```python
from build123d import *

# Parameters (mm, degrees)
CROQUIS1_W               = 70
CROQUIS1_H               = 64.6
CROQUIS1_W_2             = 50
CROQUIS1_H_2             = 44.6
SALIENTE_EXTRUIR1_DEPTH  = 5
CROQUIS2_W               = 8
CROQUIS2_H               = 5
SALIENTE_EXTRUIR2_DEPTH  = 5
REDONDEO1_R              = 0.5
REDONDEO1_OF_SIMETR_A1_R = 0.5
REDONDEO2_R              = 5


with BuildPart() as part:
    # Croquis1 → Saliente-Extruir1 (new body)
    with BuildSketch(Plane.XY):
        Rectangle(CROQUIS1_W, CROQUIS1_H)
        Rectangle(CROQUIS1_W_2, CROQUIS1_H_2, mode=Mode.SUBTRACT)
    extrude(amount=SALIENTE_EXTRUIR1_DEPTH)

    # Croquis2 → Saliente-Extruir2 (add)
    with BuildSketch(Plane.XZ.offset(32.3)):
        with Locations((-20, 2.5)):
            Rectangle(CROQUIS2_W, CROQUIS2_H)
        with Locations((20, 2.5)):
            Rectangle(CROQUIS2_W, CROQUIS2_H)
    saliente_extruir2 = extrude(amount=SALIENTE_EXTRUIR2_DEPTH)

    # Redondeo1
    redondeo1_edges = [part.edges().sort_by_distance(p)[0] for p in [
        (-24, -34.8, 5),
        (-24, -34.8, 0),
        (-16, -34.8, 0),
        (-16, -34.8, 5),
        (-24, -37.3, 2.5),
        (-20, -37.3, 0),
        (-16, -37.3, 2.5),
        (-20, -37.3, 5),
        (16, -34.8, 0),
        (24, -34.8, 0),
        (24, -34.8, 5),
        (16, -34.8, 5),
        (20, -37.3, 0),
        (24, -37.3, 2.5),
        (20, -37.3, 5),
        (16, -37.3, 2.5),
    ]]
    fillet(redondeo1_edges, radius=REDONDEO1_R)

    # Simetría1: Saliente-Extruir2 across plane
    add(saliente_extruir2.mirror(Plane.ZX))

    # Redondeo1 of Simetría1
    redondeo1_of_simetr_a1_edges = [part.edges().sort_by_distance(p)[0] for p in [
        (-24, 34.8, 5),
        (-24, 34.8, 0),
        (-16, 34.8, 0),
        (-16, 34.8, 5),
        (-24, 37.3, 2.5),
        (-20, 37.3, 0),
        (-16, 37.3, 2.5),
        (-20, 37.3, 5),
        (16, 34.8, 0),
        (24, 34.8, 0),
        (24, 34.8, 5),
        (16, 34.8, 5),
        (20, 37.3, 0),
        (24, 37.3, 2.5),
        (20, 37.3, 5),
        (16, 37.3, 2.5),
    ]]
    fillet(redondeo1_of_simetr_a1_edges, radius=REDONDEO1_OF_SIMETR_A1_R)

    # Redondeo2
    redondeo2_edges = [part.edges().sort_by_distance(p)[0] for p in [
        (-25, 22.3, 2.5),
        (-25, -22.3, 2.5),
        (25, -22.3, 2.5),
        (25, 22.3, 2.5),
        (-35, 32.3, 2.5),
        (35, 32.3, 2.5),
        (35, -32.3, 2.5),
        (-35, -32.3, 2.5),
    ]]
    fillet(redondeo2_edges, radius=REDONDEO2_R)


solid = part.part
```
The model under review builds one solid part; all positions refer to its coordinate system, in mm. A direction names the side the tool comes from. Round coordinates to 2 decimals unless told otherwise and drop trailing zeros. Write each loop counter-clockwise with the first axis right and the second up, starting at its lowest first coordinate (ties: lowest second). Pieces come first, ordered by that corner, then holes.
(1) Mouldability with a two-part tool opening along Y and no side actions: class faces 1 (the flat face through (0, -32.3, 2)), 2 (the flat face through (0, -22.3, 2)), 3 (the flat face through (16, -35, 2)) as +Y half, -Y half, draft (parallel to the pull), parting line (faces both ways), or undercut.
(2) We need section D-D on y = -31. Give the boundary of the cut face in (x, z).
(3) We need section A-A on x = 19. Give the boundary of the cut face in (y, z).
(4) Wall thickness on L1, parallel to X at y = -2.5, z = 2.75; L2, parallel to Y at x = -9.5, z = 4.85; L3, parallel to X at y = -32.5, z = 0.9: over which ranges is each line inside the solid? List them lowest first.
(5) We need section B-B on y = -7.5. Give the boundary of the cut face in (x, z), and give its area (3 significant figures).
(6) We need section C-C on x = 4. Give the boundary of the cut face in (y, z).
(7) Machinability: for faces 4 (the flat face through (-16, -35, 2)), 5 (the flat face through (-20, -37.3, 3)), 6 (the flat face through (-16, 35, 2)), 7 (the flat face through (-24, 35, 2)), 8 (the cylindrical face through (-23.5, 20.87, 2.54)), which of the approach directions +Z, -Z, +X, -X, +Y, -Y give a long, thin tool a straight path to every point of the face, cutting with its end or side? Answer none if there is none.
(8) Insertion check: pin 1 (3 mm diameter, centred on y = -35.5, z = 3.5, fed in from +X); pin 2 (2.5 mm diameter, centred on x = -7.5, z = 2, fed in from -Y); pin 3 (2.5 mm diameter, centred on x = -1.5, z = 1.5, fed in from +Y). Each pin has a flat end and moves straight along its axis. Give the tip position at first contact, or say it passes through.
Findings below:
1. face 1: -Y half
1. face 2: undercut
1. face 3: draft
2. outline: (-33.36, 0) - (33.36, 0) - (33.36, 5) - (-33.36, 5) - close
3. outline: (-37.3, 0.5) arc R0.5 ccw to (-36.8, 0) - (-22.3, 0) - (-22.3, 5) - (-36.8, 5) arc R0.5 ccw to (-37.3, 4.5) - close; (22.3, 0) - (36.8, 0) arc R0.5 ccw to (37.3, 0.5) - (37.3, 4.5) arc R0.5 ccw to (36.8, 5) - (22.3, 5) - close
4. L1: x = -35 to -25, 25 to 35
4. L2: y = -32.3 to -22.3, 22.3 to 32.3
4. L3: x = -24 to -16, 16 to 24
5. outline: (-35, 0) - (-25, 0) - (-25, 5) - (-35, 5) - close; (25, 0) - (35, 0) - (35, 5) - (25, 5) - close
5. area: 100 mm2
6. outline: (-32.3, 0) - (-22.3, 0) - (-22.3, 5) - (-32.3, 5) - close; (22.3, 0) - (32.3, 0) - (32.3, 5) - (22.3, 5) - close
7. face 4: +Z, -Z, -Y
7. face 5: +Z, -Z, +X, -X, -Y
7. face 6: +Z, -Z, +Y
7. face 7: +Z, -Z, -X, +Y
7. face 8: +Z, -Z
8. pin 1: stops at x = 24
8. pin 2: stops at y = -32.3
8. pin 3: stops at y = 32.3
